Autodesk Inventor part; units mm, degrees
ref_plane "YZ Plane" through (0, 0, 0) normal (1, 0, 0) x (0, 1, 0)
ref_plane "XZ Plane" through (0, 0, 0) normal (0, 1, 0) x (-1, 0, 0)
ref_plane "XY Plane" through (0, 0, 0) normal (0, 0, 1) x (1, 0, 0)
sketch "Sketch44" plane through (0, 0, 0) normal (0, 1, 0) x (-1, 0, 0)
  line L0 (-39.5, 120) -> (39.5, 120)
  line L1 (39.5, 120) -> (39.5, -120)
  line L2 (39.5, -120) -> (-39.5, -120)
  line L3 (-39.5, -120) -> (-39.5, 120)
  line L4 (-39.5, 120) -> (39.5, -120) construction
  line L5 (39.5, 120) -> (-39.5, -120) construction
  point P0 (0, 0)
  dimension "d138" = 79
  dimension "d139" = 240
extrude "Extrusion33" add sketch "Sketch44" along normal blind 3
sketch "Sketch45" plane through (0, 3, 0) normal (0, 1, 0) x (1, 0, 0)
  line L0 (35, -20) -> (-3, -20)
  line L1 (-3, -20) -> (-3, 20)
  line L2 (-3, 20) -> (35, 20)
  line L3 (35, 20) -> (35, -20)
  point P0 (0, 0)
  dimension "d142" = 38
  dimension "d143" = 40
extrude "Extrusion34" add sketch "Sketch45" along normal blind 30
sketch "Sketch47" plane through (0, 0, 0) normal (0, -1, 0) x (1, 0, 0)
  circle A0 centre (16, 0) radius 18
  point P0 (0, 0)
  dimension "d146" = 36
extrude "Extrusion35" cut sketch "Sketch47" against normal blind 30 draft -15
sketch "Sketch58" plane through (35, 3, -20) normal (0, 0, -1) x (-1, 0, 0)
  line L0 (7, 20) -> (27, 20)
  line L1 (27, 20) -> (27, 5)
  line L2 (27, 5) -> (7, 5)
  line L3 (7, 5) -> (7, 20)
  point P0 (35, -3)
  dimension "d156" = 20
  dimension "d157" = 15
extrude "Extrusion38" cut sketch "Sketch58" against normal blind 15
sketch "Sketch59" plane through (-3, 3, -20) normal (-1, 0, 0) x (0, 0, 1)
  line L0 (4.5, 25) -> (8, 25)
  line L1 (8, 25) -> (8, 5)
  line L2 (8, 5) -> (4.5, 5)
  line L3 (4.5, 5) -> (4.5, 25)
  point P0 (20, -3)
  dimension "d160" = 3.5
  dimension "d161" = 20
extrude "Extrusion39" cut sketch "Sketch59" against normal blind 35
sketch "Sketch60" plane through (0, 3, 0) normal (0, 1, 0) x (1, 0, 0)
  line L0 (-33.965, 38.3247) -> (-28.965, 38.3247)
  line L1 (-28.965, 38.3247) -> (-28.965, 58.3247)
  line L2 (-28.965, 58.3247) -> (-33.965, 58.3247)
  line L3 (-33.965, 58.3247) -> (-33.965, 38.3247)
  point P0 (0, 0)
  dimension "d164" = 5
  dimension "d165" = 20
extrude "Extrusion40" add sketch "Sketch60" along normal blind 20
sketch "Sketch61" plane through (0, 23, 0) normal (0, 1, 0) x (1, 0, 0)
  line L0 (-28.965, 38.3247) -> (-28.965, 58.3247)
  line L1 (-28.965, 38.3247) -> (-48.965, 38.3247)
  line L2 (-48.965, 38.3247) -> (-48.965, 58.3247)
  line L3 (-48.965, 58.3247) -> (-28.965, 58.3247)
  line L4 (-28.965, 58.3247) -> (-28.965, 38.3247)
  point P0 (0, 0)
  dimension "d168" = 20
  dimension "d169" = 20
extrude "Extrusion41" add sketch "Sketch61" against normal blind 5
sketch "Sketch65" plane through (-3, 3, -20) normal (-1, 0, 0) x (0, 0, 1)
  circle A0 centre (20, 15) radius 3
  point P0 (20, -3)
  dimension "d176" = 6
extrude "Extrusion43" cut sketch "Sketch65" against normal blind 10
sketch "Sketch68" plane through (0, 3, 0) normal (0, 1, 0) x (1, 0, 0)
  circle A0 centre (-31.5, -112) radius 3.35
  circle A1 centre (31.5, -112) radius 3.35
  circle A2 centre (-31.5, 112) radius 3.35
  circle A3 centre (31.5, 112) radius 3.35
  point P0 (0, 0)
  dimension "d192" = 6.7
  dimension "d193" = 6.7
  dimension "d194" = 6.7
  dimension "d195" = 6.7
extrude "Extrusion46" cut sketch "Sketch68" against normal through all
sketch "Sketch69" plane through (0, 3, 0) normal (0, 1, 0) x (1, 0, 0)
  circle A0 centre (23.5, -27) radius 3.35
  circle A1 centre (23.5, 27) radius 3.35
  point P0 (0, 0)
  dimension "d198" = 6.7
  dimension "d199" = 6.7
extrude "Extrusion47" cut sketch "Sketch69" against normal through all
sketch "Sketch70" plane through (0, 0, 0) normal (0, -1, 0) x (1, 0, 0)
  line L0 (-3, -12) -> (32, -12)
  line L1 (2.479, -12) -> (29.6644, -12)
  line L2 (29.6644, -12) -> (29.6644, -18.105)
  line L3 (29.6644, -18.105) -> (2.479, -18.105)
  line L4 (2.479, -18.105) -> (2.479, -12)
  point P0 (0, 0)
extrude "Extrusion48" add sketch "Sketch70" against normal blind 8
sketch "Sketch74" plane through (0, 33, 0) normal (0, 1, 0) x (1, 0, 0)
  circle A0 centre (20, 0) radius 1.15
  point P0 (0, 0)
  dimension "d210" = 2.3
extrude "Extrusion51" cut sketch "Sketch74" against normal blind 10
equation "\"d193\" = d192"
equation "\"d194\" = d192"
equation "\"d195\" = d192"
equation "\"d198\" = d192"
equation "\"d199\" = d192"
properties part number "liquid port_v10"
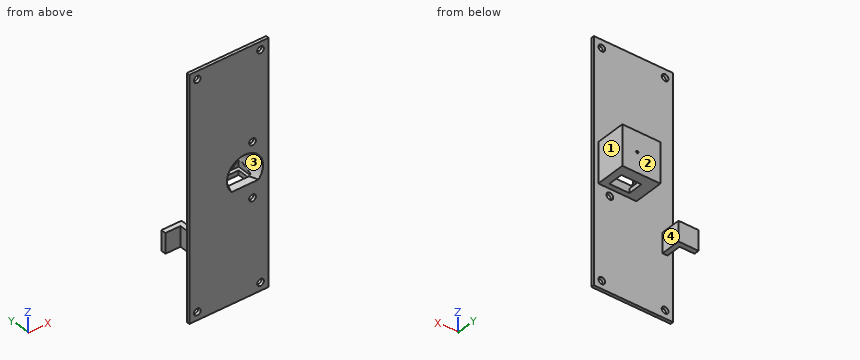
Could you check a few things on this model? Use its own coordinates, in mm. Face numbers are marked on the shaded views. A direction names the side the tool comes from. Round coordinates to 2 decimals unless told otherwise and drop trailing zeros. Loops run counter-clockwise (first coordinate to the right, second up) from the corner with the lowest first, then second, coordinate; pieces in that order, holes last.
Q1. I want a section at D-D (x = -15). Write out the boundary of the cut face in (y, z).
Q2. I want a section at C-C (z = -40.5). Write out the boundary of the cut face in (x, y) (3 decimals), and give its area (3 significant figures).
Q3. On a 3-axis mill with a long thin cutter (end or side, diameter ignored), from which of +Z, -Z, +X, -X, +Y, -Y can I reach the whole of each face in a straight line? I mean the marked faces 1 and 2. Say none if no direction works.
Q4. I want a section at A-A (z = 112). Write out the boundary of the cut face in (x, y).
Q5. Thinking about a two-plate mould opening in Z: for the marked faces 3 and 4, which applies, pulls with the +Z half, pulls with the -Z half, needs draft (parallel to the pull), parting line crosses it, or undercut?
Q6. For P1, Ø2.5, axis at x = 20, z = 0, coming from the -Y side; P2, Ø8.5, axis at x = 23.5, z = 27, coming from the +Y side; P3, Ø10, axis at x = 2.5, y = 22.5, coming from the +Z side; P4, Ø6, axis at x = 31.5, z = 112, coming from the +Y side, each with a flat end and sliding along its axis, tell me the tip position at first contact or that it passes through.
Q7. Please list where these lines run through material, in increasing order: L1, parallel to X at y = 1.1, z = -112; L2, parallel to Z at x = -31, y = 1; L3, parallel to Z at x = 31.5, y = 1.65.
Q8. I want a section at B-B (x = 16). Write out the boundary of the cut face in (y, z), and give its area (3 significant figures).
Answer below:
1. outline: (0, -120) - (3, -120) - (3, 120) - (0, 120) - close
2. outline: (-48.965, 18) - (-33.965, 18) - (-33.965, 3) - (-39.5, 3) - (-39.5, 0) - (39.5, 0) - (39.5, 3) - (-28.965, 3) - (-28.965, 23) - (-48.965, 23) - close
2. area: 412 mm2
3. face 1: +Z, -Z, +X, +Y
3. face 2: +Z, -Z, +X, -X, +Y
4. outline: (-39.5, 0) - (-34.85, 0) - (-34.85, 3) - (-39.5, 3) - close; (-28.15, 0) - (28.15, 0) - (28.15, 3) - (-28.15, 3) - close; (34.85, 0) - (39.5, 0) - (39.5, 3) - (34.85, 3) - close
5. face 3: undercut
5. face 4: needs draft
6. P1: stops at y = 30
6. P2: stops at y = 3
6. P3: stops at z = 20
6. P4: passes through
7. L1: x = -39.5 to -34.85, -28.15 to 28.15, 34.85 to 39.5
7. L2: z = -120 to -115.31, -108.69 to 108.69, 115.31 to 120
7. L3: z = -120 to -115.35, -108.65 to -8.25, 8.25 to 108.65, 115.35 to 120
8. outline: (0, -120) - (3, -120) - (3, -20) - (8, -20) - (8, -12) - (0, -12) - close; (0, 18) - (30, 9.96) - (30, -9.96) - (23, -11.84) - (23, -12) - (28, -12) - (28, -15.5) - (23, -15.5) - (23, -20) - (33, -20) - (33, 20) - (3, 20) - (3, 120) - (0, 120) - close
8. area: 1,010 mm2
